Autodesk Inventor part; units mm, degrees
ref_plane "Work Plane1" through (3.725, -0.8, 0) normal (0, 0, -1) x (-1, 0, 0)
ref_plane "YZ Plane" through (0, 0, 0) normal (1, 0, 0) x (0, 1, 0)
ref_plane "XZ Plane" through (0, 0, 0) normal (0, 1, 0) x (-1, 0, 0)
sketch "Sketch1" plane through (0, 0, 0) normal (0, 1, 0) x (-1, 0, 0)
  line L0 (3.725, 9.375) -> (-3.725, 9.375)
  line L1 (-10.6, 2.5) -> (-10.6, -2.5)
  line L2 (-3.725, -9.375) -> (3.725, -9.375)
  line L3 (10.6, -2.5) -> (10.6, 2.5)
  line L4 (16.8334, 0) -> (-16.8334, 0) construction
  line L5 (0, -15.1184) -> (0, 15.1184) construction
  arc A0 (10.6, 2.5) -> (3.725, 9.375) centre (3.725, 2.5) ccw
  arc A1 (3.725, -9.375) -> (10.6, -2.5) centre (3.725, -2.5) ccw
  arc A2 (-10.6, -2.5) -> (-3.725, -9.375) centre (-3.725, -2.5) ccw
  arc A3 (-3.725, 9.375) -> (-10.6, 2.5) centre (-3.725, 2.5) ccw
  point P0 (0, 0)
  point P1 (-10.6, -9.375)
  point P2 (-10.6, 9.375)
  point P3 (10.6, -9.375)
  dimension "d0" = 21.2
  dimension "d1" = 18.75
  dimension "d2" = 6.875
extrude "Extrusion1" add sketch "Sketch1" against normal blind 0.8
sketch "Sketch2" plane through (0, -0.8, 0) normal (0, -1, 0) x (1, 0, 0)
  line L0 (10.6, -2.5) -> (10.6, 2.5)
  arc A0 (10.6, 2.5) -> (3.725, 9.375) centre (3.725, 2.5) ccw
  arc A1 (3.725, -9.375) -> (10.6, -2.5) centre (3.725, -2.5) ccw
  line L1 (-3.725, -9.375) -> (3.725, -9.375)
  arc A2 (-10.6, -2.5) -> (-3.725, -9.375) centre (-3.725, -2.5) ccw
  line L2 (-10.6, 2.5) -> (-10.6, -2.5)
  arc A3 (-3.725, 9.375) -> (-10.6, 2.5) centre (-3.725, 2.5) ccw
  line L3 (3.725, 9.375) -> (-3.725, 9.375)
  arc A4 (10, 2.5) -> (3.725, 8.775) centre (3.725, 2.5) ccw
  line L4 (10, 2.5) -> (10, -2.5)
  arc A5 (3.725, -8.775) -> (10, -2.5) centre (3.725, -2.5) ccw
  line L5 (3.725, -8.775) -> (-3.725, -8.775)
  arc A6 (-10, -2.5) -> (-3.725, -8.775) centre (-3.725, -2.5) ccw
  line L6 (-10, -2.5) -> (-10, 2.5)
  arc A7 (-3.725, 8.775) -> (-10, 2.5) centre (-3.725, 2.5) ccw
  line L7 (-3.725, 8.775) -> (3.725, 8.775)
  arc A8 (8.25, 2.5) -> (3.725, 7.025) centre (3.725, 2.5) ccw
  line L8 (8.25, 2.5) -> (8.25, -2.5)
  arc A9 (3.725, -7.025) -> (8.25, -2.5) centre (3.725, -2.5) ccw
  line L9 (3.725, -7.025) -> (-3.725, -7.025)
  arc A10 (-8.25, -2.5) -> (-3.725, -7.025) centre (-3.725, -2.5) ccw
  line L10 (-8.25, -2.5) -> (-8.25, 2.5)
  arc A11 (-3.725, 7.025) -> (-8.25, 2.5) centre (-3.725, 2.5) ccw
  line L11 (-3.725, 7.025) -> (3.725, 7.025)
  arc A12 (7.65, 2.5) -> (3.725, 6.425) centre (3.725, 2.5) ccw
  line L12 (7.65, 2.5) -> (7.65, -2.5)
  arc A13 (3.725, -6.425) -> (7.65, -2.5) centre (3.725, -2.5) ccw
  line L13 (3.725, -6.425) -> (-3.725, -6.425)
  arc A14 (-7.65, -2.5) -> (-3.725, -6.425) centre (-3.725, -2.5) ccw
  line L14 (-7.65, -2.5) -> (-7.65, 2.5)
  arc A15 (-3.725, 6.425) -> (-7.65, 2.5) centre (-3.725, 2.5) ccw
  line L15 (-3.725, 6.425) -> (3.725, 6.425)
  arc A16 (5.9, 2.5) -> (3.725, 4.675) centre (3.725, 2.5) ccw
  line L16 (5.9, 2.5) -> (5.9, -2.5)
  arc A17 (3.725, -4.675) -> (5.9, -2.5) centre (3.725, -2.5) ccw
  line L17 (3.725, -4.675) -> (-3.725, -4.675)
  arc A18 (-5.9, -2.5) -> (-3.725, -4.675) centre (-3.725, -2.5) ccw
  line L18 (-5.9, -2.5) -> (-5.9, 2.5)
  arc A19 (-3.725, 4.675) -> (-5.9, 2.5) centre (-3.725, 2.5) ccw
  line L19 (-3.725, 4.675) -> (3.725, 4.675)
  arc A20 (5.3, 2.5) -> (3.725, 4.075) centre (3.725, 2.5) ccw
  line L20 (5.3, 2.5) -> (5.3, -2.5)
  arc A21 (3.725, -4.075) -> (5.3, -2.5) centre (3.725, -2.5) ccw
  line L21 (3.725, -4.075) -> (-3.725, -4.075)
  arc A22 (-5.3, -2.5) -> (-3.725, -4.075) centre (-3.725, -2.5) ccw
  line L22 (-5.3, -2.5) -> (-5.3, 2.5)
  arc A23 (-3.725, 4.075) -> (-5.3, 2.5) centre (-3.725, 2.5) ccw
  line L23 (-3.725, 4.075) -> (3.725, 4.075)
  line L24 (3.725, 4.075) -> (3.725, 4.675)
  line L25 (3.725, -4.075) -> (3.725, -4.675)
  point P0 (0, 0)
  dimension "d5" = 0.6
  dimension "d6" = 1.75
  dimension "d7" = 0.6
  dimension "d8" = 1.75
  dimension "d9" = 0.6
extrude "Extrusion2" add sketch "Sketch2" along normal blind 1.1 contours A1 L1 A2 L2 A3 L3 A0 L0 | L8 A9 L9 A10 L10 A11 L11 A8 | L24 L23 A23 L22 A22 L21 L25 L17 A18 L18 A19 L19
sketch "Sketch3" plane through (0, 0, 0) normal (0, 1, 0) x (1, 0, 0)
  line L0 (7.95, 4.3) -> (-8.65, 4.3)
  line L1 (-8.65, 4.3) -> (-8.65, -4.3)
  line L2 (-8.65, -4.3) -> (7.95, -4.3)
  line L3 (7.95, -4.3) -> (7.95, 4.3)
  line L4 (-14.84, 0) -> (14.84, 0) construction
  line L5 (-10.6, 2.5) -> (-10.6, -2.5)
  point P0 (0, 0)
  dimension "d12" = 16.6
  dimension "d13" = 8.6
  dimension "d14" = 1.95
extrude "Extrusion3" add sketch "Sketch3" along normal blind 2.8
sketch "Sketch4" plane through (0, 2.8, 0) normal (0, 1, 0) x (1, 0, 0)
  line L0 (0.7, 2.3) -> (-5.5, 2.3)
  line L1 (-5.5, 2.3) -> (-5.5, -2.3)
  line L2 (-5.5, -2.3) -> (0.7, -2.3)
  line L3 (0.7, -2.3) -> (0.7, 2.3)
  line L4 (-14.84, 0) -> (14.84, 0) construction
  line L5 (-8.65, 4.3) -> (-8.65, -4.3)
  point P0 (0, 0)
  dimension "d17" = 6.2
  dimension "d18" = 4.6
  dimension "d19" = 3.15
extrude "Extrusion4" cut sketch "Sketch4" against normal blind 2.1
sketch "Sketch5" plane through (0, 2.8, 0) normal (0, 1, 0) x (1, 0, 0)
  line L0 (-8.65, 4.3) -> (7.95, 4.3)
  line L1 (7.95, 4.3) -> (5.15, 4.3)
  line L2 (5.15, 4.3) -> (5.15, 2.7)
  line L3 (5.15, 2.7) -> (7.95, 2.7)
  line L4 (7.95, 2.7) -> (7.95, 4.3)
  line L5 (-8.65, -4.3) -> (7.95, -4.3)
  line L6 (7.95, -4.3) -> (5.15, -4.3)
  line L7 (5.15, -4.3) -> (5.15, -2.7)
  line L8 (5.15, -2.7) -> (7.95, -2.7)
  line L9 (7.95, -2.7) -> (7.95, -4.3)
  line L10 (-8.65, 4.3) -> (-8.65, -4.3)
  line L11 (-8.65, -4.3) -> (-6.9, -4.3)
  line L12 (-6.9, -4.3) -> (-6.9, -2.9)
  line L13 (-6.9, -2.9) -> (-8.65, -2.9)
  line L14 (-8.65, -2.9) -> (-8.65, -4.3)
  line L15 (-8.65, 4.3) -> (-6.9, 4.3)
  line L16 (-6.9, 4.3) -> (-6.9, 2.9)
  line L17 (-6.9, 2.9) -> (-8.65, 2.9)
  line L18 (-8.65, 2.9) -> (-8.65, 4.3)
  point P0 (0, 0)
  dimension "d22" = 2.8
  dimension "d23" = 1.6
  dimension "d24" = 2.8
  dimension "d25" = 1.6
  dimension "d26" = 1.75
  dimension "d27" = 1.4
  dimension "d28" = 1.75
  dimension "d29" = 1.4
extrude "Extrusion5" add sketch "Sketch5" along normal blind 1.9
sketch "Sketch6" plane through (0, 0, 0) normal (0, 1, 0) x (1, 0, 0)
  arc A0 (-3.725, 9.375) -> (-10.6, 2.5) centre (-3.725, 2.5) ccw
  line L0 (-8.65, -4.3) -> (-8.65, 4.3)
  line L1 (-10.6, 2.5) -> (-8.65, 2.5)
  line L2 (-8.65, 2.5) -> (-8.65, -2.5)
  line L3 (-8.65, -2.5) -> (-10.6, -2.5)
  line L4 (-10.6, -2.5) -> (-10.6, 2.5)
  line L5 (10.6, 2.5) -> (10.6, -2.5)
  line L6 (7.95, 4.3) -> (7.95, -4.3)
  line L7 (10.6, 2.5) -> (7.95, 2.5)
  line L8 (7.95, 2.5) -> (7.95, -2.5)
  line L9 (7.95, -2.5) -> (10.6, -2.5)
  line L10 (10.6, -2.5) -> (10.6, 2.5)
  point P0 (0, 0)
  dimension "d32" = 5
  dimension "d33" = 5
extrude "Extrusion6" add sketch "Sketch6" along normal blind 1
sketch "Sketch7" plane through (0, 4.7, 0) normal (0, 1, 0) x (1, 0, 0)
  circle A0 centre (5.9, 3.415) radius 0.45
  circle A1 centre (-7.64, -3.415) radius 0.45
  line L0 (5.15, 4.3) -> (5.15, 2.7)
  line L1 (-6.9, -4.3) -> (-6.9, -2.9)
  line L2 (5.15, 2.7) -> (7.95, 2.7)
  line L3 (-6.9, -2.9) -> (-8.65, -2.9)
  point P0 (0, 0)
  point P1 (5.15, 3.5)
  point P2 (-6.9, -3.6)
  point P3 (6.55, 2.7)
  point P4 (-7.775, -2.9)
  dimension "d36" = 0.9
  dimension "d37" = 0.9
  dimension "d48" = 13.54
  dimension "d49" = 6.83
  dimension "d50" = 3.415
  dimension "d52" = 5.9
extrude "Extrusion7" add sketch "Sketch7" along normal blind 1.75
ref_plane "Work Plane1" through (3.725, -0.8, 0) normal (0, 0, -1) x (-1, 0, 0)
sketch "Sketch8" plane through (3.725, -0.8, 0) normal (0, 0, -1) x (-1, 0, 0)
  line L0 (0, 0) -> (0, -1.1) construction
  line L1 (1.5943, 0) -> (0, -1.9)
  line L2 (0, -1.9) -> (-0.6915, 0)
  line L3 (7.45, -1.1) -> (0, -1.1) construction
  line L4 (0, 0) -> (7.45, 0)
  line L5 (-3.925, 0) -> (0, 0)
  point P0 (3.725, 0.8)
  dimension "d40" = 0.8
  dimension "d41" = 60
  dimension "d42" = 70
extrude "Extrusion8" add sketch "Sketch8" along normal mid plane 4
sketch "Sketch9" plane through (0, -0.8, 0) normal (0, -1, 0) x (1, 0, 0)
  circle A0 centre (-1.225, 0) radius 1.375
  arc A1 (-3.725, 4.075) -> (-5.3, 2.5) centre (-3.725, 2.5) ccw
  arc A2 (-5.3, -2.5) -> (-3.725, -4.075) centre (-3.725, -2.5) ccw
  line L0 (-3.725, 2.5) -> (-1.225, 0) construction
  line L1 (-1.225, 0) -> (-3.725, -2.5) construction
  point P0 (0, 0)
  dimension "d45" = 2.75
extrude "Extrusion9" add sketch "Sketch9" along normal blind 0.2
equation "\"d29\" = d27"
properties part number "LM19-LSI_lens" material "Polycarbonate, Clear"
Geometry check sheet. Reference: the model listing, model coordinates, mm. A direction names the side the tool comes from. Round coordinates to 2 decimals unless told otherwise and drop trailing zeros. Order: outer loops, then holes, each group sorted by start corner. A loop starts at its lowest first (then second) coordinate and runs counter-clockwise, first axis right, second up. Notation, with made-up numbers: M 61,73.5 L 65,73.5 A20 cw 65,90.5 Z; hole C -10,-39.5 d11. An arc over 180 degrees is marked long. Write each question's results on one line, items separated by ' | '. Start each with the question number.
1. Cross-section at A-A on y = 1.75. Record the boundary of the cut face in (x, z), plus the area to 3 significant figures.
2. Cross-section at C-C on x = 1.25. Record the boundary of the cut face in (y, z) (3 decimals), plus the area to 3 significant figures.
3. Cross-section at D-D on z = -5.75. Record the boundary of the cut face in (x, y).
4. Cross-section at B-B on y = -0.5. Record the boundary of the cut face in (x, z) (3 decimals).
5. Go/stop test with flat-tipped pins: P1, Ø1.5, axis at x = 8.5, y = 0, coming from the +Z side; P2, Ø0.8, axis at x = 9, z = -0.5, coming from the +Y side; P3, Ø0.8, axis at x = -9.5, y = 0.5, coming from the +Z side. Record where each tip stops, or that it passes through.
6. Set-up check for faces 1 (the face through (-2, 2, 2.3)), 2 (the face through (0, -1, -8.775)), 3 (the face through (0, 2, -4.3)), 4 (the face through (0, 2, 4.3)), 5 (the face through (5.15, 4, 4)): record each of +Z, -Z, +X, -X, +Y, -Y from which the full face is reachable in a straight line by a thin tool's end or side.
7. Material ranges on L1, parallel to Y at x = -0.5, z = -5.25; L2, parallel to Y at x = 1, z = -0.25; L3, parallel to X at y = -1.5, z = -3, recorded low to high. Write a range as from..to.
8. Draft check along X on faces 6 (the face through (7, 4.7, 3)), 7 (the face through (-8.64, -0.937, 7.308)), 8 (the face through (10, -1, 0)). Enter one of: pulls with the +X half, pulls with the -X half, needs draft (parallel to the pull), parting line crosses it, or undercut.
Resolved:
1) outline: M -8.65,-4.3 L 7.95,-4.3 L 7.95,4.3 L -8.65,4.3 Z; hole M -5.5,-2.3 L 0.7,-2.3 L 0.7,2.3 L -5.5,2.3 Z | area: 114 mm2
2) outline: M -1.9,-9.375 L 0,-9.375 L 0,-4.3 L 2.8,-4.3 L 2.8,4.3 L 0,4.3 L 0,9.375 L -1.9,9.375 L -1.9,8.775 L -0.8,8.775 L -0.8,7.025 L -1.9,7.025 L -1.9,6.425 L -0.8,6.425 L -0.8,4.675 L -1.9,4.675 L -1.9,4.075 L -0.8,4.075 L -0.8,-4.075 L -1.9,-4.075 L -1.9,-4.675 L -0.8,-4.675 L -0.8,-6.425 L -1.9,-6.425 L -1.9,-7.025 L -0.8,-7.025 L -0.8,-8.775 L -1.9,-8.775 Z | area: 43.0 mm2
3) outline: M -9.78,-1.9 L -9.09,-1.9 L -9.09,-0.8 L -6.87,-0.8 L -6.87,-1.9 L -5.93,-1.9 L -5.93,-0.8 L 5.93,-0.8 L 5.93,-1.9 L 6.87,-1.9 L 6.87,-0.8 L 9.09,-0.8 L 9.09,-1.9 L 9.78,-1.9 L 9.78,0 L -9.78,0 Z
4) outline: M -10.6,-2.5 A6.875 ccw -3.725,-9.375 L 3.725,-9.375 A6.875 ccw 10.6,-2.5 L 10.6,2.5 A6.875 ccw 3.725,9.375 L -3.725,9.375 A6.875 ccw -10.6,2.5 Z
5) P1: z = 8.07 | P2: y = 1 | P3: z = 2.5
6) face 1: +Y | face 2: -Y | face 3: -Z, +X, -X, +Y | face 4: +Z, +X, -X, +Y | face 5: +Z, -Z, +Y
7) L1: -0.8..0 | L2: -0.8..2.8 | L3: -10.58..-9.98, -8.22..-7.62, -5.84..-5.22, 7.62..8.22, 9.98..10.58
8) face 6: needs draft | face 7: pulls with the -X half | face 8: undercut
